Drawing for the job (mm, zero at the part's lowest x, y, z). Give positions to 0.01 mm unless a question says otherwise; leave off trailing zeros. Order: outer loops, then holes, each group sorted by start corner. A loop starts at its lowest first (then second) coordinate and runs counter-clockwise, first axis right, second up. Notation, with made-up numbers: (6, -9.75) -> (17, -9.75) arc R24 ccw to (17, 19.25) -> close; hole circle Ø8 at (-34.75, 19). An arc over 180 degrees is marked (long way). One line per item, written item: value. Start each with the question number.
(1) Two-plate mould, pull along Y, no slides. Class the marked faces 1, 2, 3 and 4: +Y half, -Y half, draft (parallel to the pull), parting line (faces both ways), or undercut.
(2) Saw through at B-B on y = 10. Give the cut face in (x, z), plus the area to 3 significant figures.
(3) Saw through at C-C on x = 12.5. Give the cut face in (y, z).
(4) Saw through at A-A on z = 5. Give the cut face in (x, y), plus the area to 3 significant figures.
(5) Saw through at D-D on y = 60. Give the cut face in (x, z).
(6) Probe line 1 (Y direction, x = 12.5, z = 3.75); line 2 (X direction, y = 8.5, z = 8.25); line 3 (Z direction, x = 20.75, y = 60). List the from-to ranges inside material, lowest first.
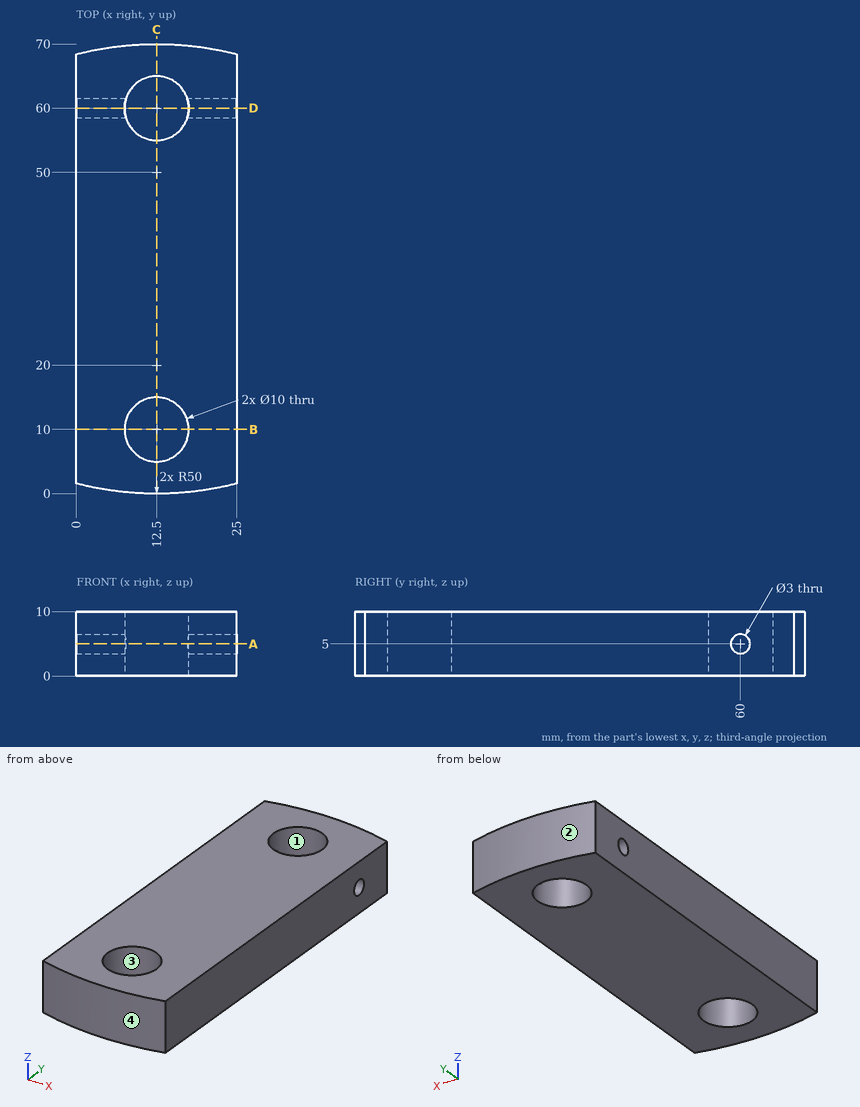
Results below:
1. face 1: undercut
1. face 2: +Y half
1. face 3: undercut
1. face 4: -Y half
2. outline: (0, 0) -> (7.5, 0) -> (7.5, 10) -> (0, 10) -> close; (17.5, 0) -> (25, 0) -> (25, 10) -> (17.5, 10) -> close
2. area: 150 mm²
3. outline: (0, 0) -> (5, 0) -> (5, 10) -> (0, 10) -> close; (15, 0) -> (55, 0) -> (55, 10) -> (15, 10) -> close; (65, 0) -> (70, 0) -> (70, 10) -> (65, 10) -> close
4. outline: (0, 1.59) arc R50 ccw to (25, 1.59) -> (25, 58.5) -> (17.27, 58.5) arc R5 cw to (7.73, 58.5) -> (0, 58.5) -> close; (0, 61.5) -> (7.73, 61.5) arc R5 cw to (17.27, 61.5) -> (25, 61.5) -> (25, 68.41) arc R50 ccw to (0, 68.41) -> close; hole circle Ø10 at (12.5, 10)
4. area: 1,520 mm²
5. outline: (0, 0) -> (7.5, 0) -> (7.5, 3.5) -> (0, 3.5) -> close; (0, 6.5) -> (7.5, 6.5) -> (7.5, 10) -> (0, 10) -> close; (17.5, 0) -> (25, 0) -> (25, 3.5) -> (17.5, 3.5) -> close; (17.5, 6.5) -> (25, 6.5) -> (25, 10) -> (17.5, 10) -> close
6. line 1: y = 0 to 5, 15 to 55, 65 to 70
6. line 2: x = 0 to 7.73, 17.27 to 25
6. line 3: z = 0 to 3.5, 6.5 to 10
